Verification items for this drawing (mm, ordinates from the low corner). A direction names the side the tool comes from. Round coordinates to 2 decimals unless told otherwise and drop trailing zeros. Order: outer loops, then holes, each group sorted by start corner. A loop starts at its lowest first (then second) coordinate and runs counter-clockwise, first axis right, second up. Notation, with made-up numbers: (67, -14.5) -> (72, -14.5) arc R20 cw to (72, 10.5) -> close; hole circle Ø1 at (-30, 34.25). An arc over 180 degrees is marked (long way). Answer in a Markdown table with one row per item. Add a question column.
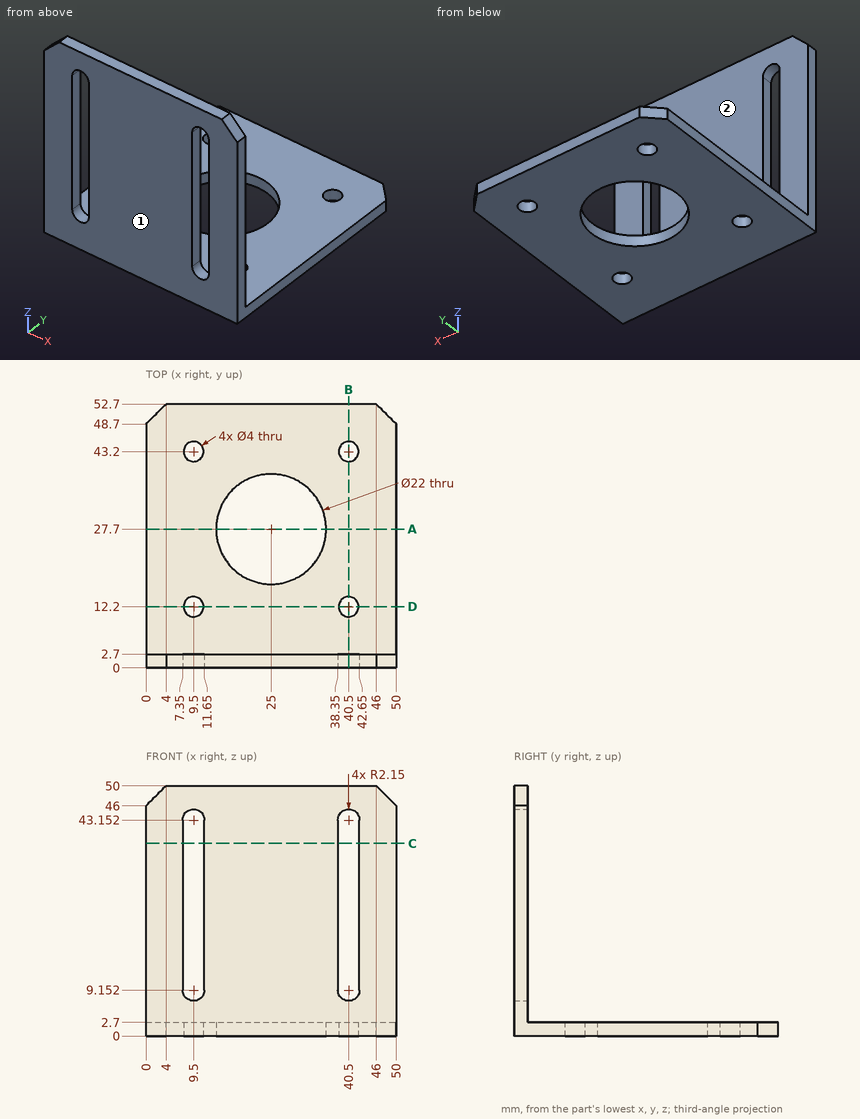
1) Cross-section at D-D, the plane y = 12.2. Record the boundary of the cut face in (x, z), and give its area (3 significant figures).
2) Cross-section at B-B, the plane x = 40.5. Record the boundary of the cut face in (y, z), and give its area (3 significant figures).
3) Tool access check on the marked faces 1 and 2. Record the directions out of +Z, -Z, +X, -X, +Y, -Y that give a thin tool (end or side, any length) a straight path to the whole face; none if there is none.
4) Thickness scan on L1, parallel to X at y = 2, z = 38; L2, parallel to X at y = 43.2, z = 1.95; L3, parallel to Z at x = 12.5, y = 5.5. Record the ranges inside material, lowest first. Write a range as [from, to].
5) Depth check by flat-ended pin: P1, Ø10, axis at x = 34, z = 14, coming from the +Y side; P2, Ø13, axis at x = 25, y = 27.7, coming from the -Z side; P3, Ø5, axis at x = 9.5, y = 43.2, coming from the +Z side; P4, Ø0.8, axis at y = 1, z = 18, coming from the -X side. Enter the tip coordinate at first touch or a pass-through.
6) Cross-section at C-C, the plane z = 38.5. Record the boundary of the cut face in (x, y), and give its area (3 significant figures).
7) Cross-section at A-A, the plane y = 27.7. Record the boundary of the cut face in (x, z).
Results below:
| question | item | result |
|---|---|---|
| 1 | outline | (0, 0) -> (7.5, 0) -> (7.5, 2.7) -> (0, 2.7) -> close; (11.5, 0) -> (38.5, 0) -> (38.5, 2.7) -> (11.5, 2.7) -> close; (42.5, 0) -> (50, 0) -> (50, 2.7) -> (42.5, 2.7) -> close |
| 1 | area | 113 mm² |
| 2 | outline | (0, 0) -> (10.2, 0) -> (10.2, 2.7) -> (2.7, 2.7) -> (2.7, 7) -> (0, 7) -> close; (0, 45.3) -> (2.7, 45.3) -> (2.7, 50) -> (0, 50) -> close; (14.2, 0) -> (41.2, 0) -> (41.2, 2.7) -> (14.2, 2.7) -> close; (45.2, 0) -> (52.7, 0) -> (52.7, 2.7) -> (45.2, 2.7) -> close |
| 2 | area | 145 mm² |
| 3 | face 1 | +Z, -Z, +X, -X, -Y |
| 3 | face 2 | +Z, +X, -X, +Y |
| 4 | L1 | [0, 7.35], [11.65, 38.35], [42.65, 50] |
| 4 | L2 | [0, 7.5], [11.5, 38.5], [42.5, 50] |
| 4 | L3 | [0, 2.7] |
| 5 | P1 | y = 2.7 |
| 5 | P2 | through |
| 5 | P3 | z = 2.7 |
| 5 | P4 | x = 0 |
| 6 | outline | (0, 0) -> (7.35, 0) -> (7.35, 2.7) -> (0, 2.7) -> close; (11.65, 0) -> (38.35, 0) -> (38.35, 2.7) -> (11.65, 2.7) -> close; (42.65, 0) -> (50, 0) -> (50, 2.7) -> (42.65, 2.7) -> close |
| 6 | area | 112 mm² |
| 7 | outline | (0, 0) -> (14, 0) -> (14, 2.7) -> (0, 2.7) -> close; (36, 0) -> (50, 0) -> (50, 2.7) -> (36, 2.7) -> close |
